from build123d import *

# Parameters (mm, degrees)
EXTRUDE_1_DEPTH     = 10
EXTRUDE_START       = 10
EXTRUDE_2_DEPTH     = 10
EXTRUDE_START_2     = -20
SKETCH_5_W          = 47.76055714
SKETCH_5_H          = 4.8
EXTRUDE_3_DEPTH     = 20
SKETCH_4_R          = 1.7
CUT_EXTRUDE_1_DEPTH = 70.746966001
EXTRUDE_1_2_DEPTH   = 245
CUT_EXTRUDE_2_DEPTH = 267.572630949
SKETCH_8_W          = 87.68405268
SKETCH_8_H          = 11.060470773
EXTRUDE_2_2_DEPTH   = 10


with BuildPart() as part:
    # 草图2 → Extrude 1 (new body)
    with BuildSketch(Plane.ZY.offset(10)):
        with BuildLine():
            ThreePointArc((17.754161429, 46.104597493), (0, 49.404900142), (-17.754161429, 46.104597493))
            Line((-17.754161429, 46.104597493), (-22.425845774, 58.236182937))
            ThreePointArc((-22.425845774, 58.236182937), (0, 62.404900142), (22.425845774, 58.236182937))
            Line((22.425845774, 58.236182937), (17.754161429, 46.104597493))
        make_face()
    extrude(amount=EXTRUDE_1_DEPTH)

    # 草图3 → Extrude 2 (add)
    with BuildSketch(Plane(origin=(-10, 0, 0), x_dir=(0, 0, -1), z_dir=(1, 0, 0)).offset(EXTRUDE_START)):
        with BuildLine():
            ThreePointArc((22.425845774, 58.236182937), (0, 62.404900142), (-22.425845774, 58.236182937))
            Line((-22.425845774, 58.236182937), (-20.700916169, 53.756828311))
            ThreePointArc((-20.700916169, 53.756828311), (0, 57.604900142), (20.700916169, 53.756828311))
            Line((20.700916169, 53.756828311), (22.425845774, 58.236182937))
        make_face()
    extrude(amount=-EXTRUDE_2_DEPTH)

    # 草图5 → 拉伸-薄壁3 (add)
    with BuildSketch(Plane(origin=(0, 0, 0), x_dir=(0, 0, -1), z_dir=(1, 0, 0)).offset(EXTRUDE_START_2)):
        with Locations((0, 60.004900142)):
            Rectangle(SKETCH_5_W, SKETCH_5_H)
    extrude(amount=EXTRUDE_3_DEPTH)

    # 草图4 → 切除-拉伸1 (cut, through all)
    with BuildSketch(Plane(origin=(0, 0, 0), x_dir=(1, 0, 0), z_dir=(0, 1, 0))):
        with Locations(Location((-4.960065679, 0, 0), (0, 0, 90))):
            Circle(SKETCH_4_R)
    extrude(amount=CUT_EXTRUDE_1_DEPTH, mode=Mode.SUBTRACT)

    # 草图6 → Extrude 1 2 (add)
    with BuildSketch(Plane.ZY.offset(20)):
        with BuildLine():
            Line((23.88027857, 62.404900142), (-23.88027857, 62.404900142))
            Line((-23.88027857, 62.404900142), (-23.88027857, 57.604900142))
            Line((-23.88027857, 57.604900142), (-22.182748615, 57.604900142))
            Line((-22.182748615, 57.604900142), (-17.754161429, 46.104597493))
            ThreePointArc((-17.754161429, 46.104597493), (0, 49.404900142), (17.754161429, 46.104597493))
            Line((17.754161429, 46.104597493), (22.182748615, 57.604900142))
            Line((22.182748615, 57.604900142), (23.88027857, 57.604900142))
            Line((23.88027857, 57.604900142), (23.88027857, 62.404900142))
        make_face()
    extrude(amount=EXTRUDE_1_2_DEPTH)

    # 草图7 → 切除-拉伸2 (cut, through all)
    with BuildSketch(Plane(origin=(0, 62.404900142, 0), x_dir=(1, 0, 0), z_dir=(0, 1, 0))):
        with BuildLine():
            Line((-35.208375229, 23.88027857), (-35.208375229, 18))
            ThreePointArc((-35.208375229, 18), (-37.55152098, 12.343145751), (-43.208375229, 10))
            Line((-43.208375229, 10), (-265, 10))
            Line((-265, 10), (-265, 23.88027857))
            Line((-265, 23.88027857), (-35.208375229, 23.88027857))
        make_face()
        with BuildLine():
            Line((-43.208375229, -10), (-265, -10))
            Line((-265, -10), (-265, -23.88027857))
            Line((-265, -23.88027857), (-35.208375229, -23.88027857))
            Line((-35.208375229, -23.88027857), (-35.208375229, -18))
            ThreePointArc((-35.208375229, -18), (-37.55152098, -12.343145751), (-43.208375229, -10))
        make_face()
    extrude(amount=-CUT_EXTRUDE_2_DEPTH, mode=Mode.SUBTRACT)

    # 草图8 → Extrude 2 2 (add)
    with BuildSketch(Plane.ZY.offset(265)):
        with Locations((1.006520642, 56.874664756)):
            Rectangle(SKETCH_8_W, SKETCH_8_H)
    extrude(amount=-EXTRUDE_2_2_DEPTH)


solid = part.part
The listing builds one solid part. Answer for the finished solid, in the listing's coordinates (mm). A direction names the side the tool comes from. Give positions to 0.01 mm unless a question says otherwise; leave off trailing zeros. Loops run counter-clockwise (first coordinate to the right, second up) from the corner with the lowest first, then second, coordinate; pieces in that order, holes last.
Item 1: Determine the mould class of faces 1 (the flat face through (-260, 51.344, -27)), 2 (the flat face through (-265, 57, 0)), 3 (the flat face through (-255, 57, -27)), 4 (the flat face through (-255, 57, 27)) for opening direction X: +X half, -X half, draft (parallel to the pull), parting line (faces both ways), or undercut.
Derived:
face 1: draft
face 2: -X half
face 3: undercut
face 4: undercut
Item 2: A cutting plane is placed at C-C (y = 60). Give the vertices of the cut face in (x, z).
Derived:
outline: (-265, -42.84) - (-255, -42.84) - (-255, -10) - (-43.21, -10) arc R8 cw to (-35.21, -18) - (-35.21, -23.88) - (0, -23.88) - (0, 23.88) - (-35.21, 23.88) - (-35.21, 18) arc R8 cw to (-43.21, 10) - (-255, 10) - (-255, 44.85) - (-265, 44.85) - close; hole circle Ø3.4 at (-4.96, 0)
Item 3: Find the intervals of material crossed by line 1 along X through (y, z) = (59.15, 0); line 2 along X through (y, z) = (58.5, -19.5); line 3 along X through (y, z) = (48.25, -17.5), in increasing order.
Derived:
line 1: x = -265 to -6.66, -3.26 to 0
line 2: x = -265 to -255, -35.21 to 0
line 3: x = -35.22 to -10
Item 4: A cutting plane is placed at B-B (x = -28). Give the vertices of the cut face in (y, z).
Derived:
outline: (46.1, -17.75) - (57.6, -22.18) - (57.6, -23.88) - (62.4, -23.88) - (62.4, 23.88) - (57.6, 23.88) - (57.6, 22.18) - (46.1, 17.75) arc R49.4 cw to start
Item 5: Each of these flat-tipped pins is pushed along its axis until it touches: pin 1 Ø4 at (y, z) = (51.5, -28.5) entering from +X; pin 2 Ø5 at (x, y) = (-198, 56) entering from +Z; pin 3 Ø1.4 at (x, z) = (-14, 23.5) entering from -Y; pin 4 Ø2 at (x, z) = (-4.96, 0) entering from -Y. Where does it stop, or does it pass through?
Derived:
pin 1: stops at x = -255
pin 2: stops at z = 10
pin 3: stops at y = 57.6
pin 4: passes through
Item 6: A cutting plane is placed at A-A (z = 13). Give the vertices of the cut face in (x, y), then the cut area to 3 significant figures.
Derived:
outline: (-265, 51.34) - (-255, 51.34) - (-255, 62.4) - (-265, 62.4) - close; (-36.96, 47.66) - (-10, 47.66) - (-10, 56.12) - (0, 56.12) - (0, 62.4) - (-36.96, 62.4) - close
area: 571 mm2
Item 7: A tool of negligible diameter and unlimited length cuts with its end or side. For faces 5 (the flat face through (-35.208, 56, -20)), 6 (the flat face through (-17, 60, 23.88)), 7 (the flat face through (-35.208, 56, 20)), 8 (the cylindrical face through (-2.708, 57.604, 0.296)), from which of +Z, -Z, +X, -X, +Y, -Y can it reach the whole face along a straight path? Write none if from no direction.
Derived:
face 5: -Z, +Y, -Y
face 6: +Z, +X, +Y, -Y
face 7: +Z, +Y, -Y
face 8: +X, -Y
Item 8: A cutting plane is placed at D-D (z = -37). Give the vertices of the cut face in (x, y), then the cut area to 3 significant figures.
Derived:
outline: (-265, 51.34) - (-255, 51.34) - (-255, 62.4) - (-265, 62.4) - close
area: 111 mm2
